from build123d import *

# Parameters (mm, degrees)
SKETCH_W        = 75
SKETCH_H        = 54
PAD_DEPTH       = 10
SKETCH001_R     = 17
POCKET_DEPTH    = 7
SKETCH002_W     = 111.709
SKETCH002_H     = 38.0948
POCKET001_DEPTH = 7
SKETCH003_R     = 2
POCKET002_DEPTH = 10.001
FILLET_R        = 10
CHAMFER_SIZE    = 0.5
CHAMFER001_SIZE = 1.5


with BuildPart() as part:
    # Sketch → Pad (new body)
    with BuildSketch(Plane.XY):
        with Locations((0, 7)):
            Rectangle(SKETCH_W, SKETCH_H)
    extrude(amount=PAD_DEPTH)

    # Sketch001 → Pocket (cut)
    with BuildSketch(Plane.XY.offset(10)):
        with Locations((-18, 0)):
            Circle(SKETCH001_R)
        with Locations((18, 0)):
            Circle(SKETCH001_R)
    extrude(amount=-POCKET_DEPTH, mode=Mode.SUBTRACT)

    # Sketch002 → Pocket001 (cut)
    with BuildSketch(Plane.XY.offset(10)):
        with Locations((0, 19.0474)):
            Rectangle(SKETCH002_W, SKETCH002_H)
    extrude(amount=-POCKET001_DEPTH, mode=Mode.SUBTRACT)

    # Sketch003 → Pocket002 (cut, through all)
    with BuildSketch(Plane.XY.offset(10)):
        with Locations((-18, 0)):
            Circle(SKETCH003_R)
        with Locations((18, 0)):
            Circle(SKETCH003_R)
    extrude(amount=-POCKET002_DEPTH, mode=Mode.SUBTRACT)

    # Fillet
    fillet_edges = [part.edges().sort_by_distance(p)[0] for p in [
        (37.5, 34, 1.5),
        (-37.5, 34, 1.5),
        (-37.5, -20, 5),
        (37.5, -20, 5),
    ]]
    fillet(fillet_edges, radius=FILLET_R)

    # Chamfer
    chamfer_edges = [part.edges().sort_by_distance(p)[0] for p in [
        (-37.5, -5, 10),
        (-34.571068, -17.071068, 10),
        (-36.25, 0, 10),
        (0, -20, 10),
        (-18, -17, 10),
        (34.571068, -17.071068, 10),
        (0, 0, 10),
        (37.5, -5, 10),
        (18, -17, 10),
        (36.25, 0, 10),
    ]]
    chamfer(chamfer_edges, length=CHAMFER_SIZE)

    # Chamfer001
    chamfer001_edges = [part.edges().sort_by_distance(p)[0] for p in [
        (18, -2, 3),
        (-18, -2, 3),
    ]]
    chamfer(chamfer001_edges, length=CHAMFER001_SIZE)


solid = part.part
Model file for the job. Use its own axes, mm. A direction names the side the tool comes from. Give positions to 0.01 mm unless a question says otherwise; leave off trailing zeros. Write each loop counter-clockwise with the first axis right and the second up, starting at its lowest first coordinate (ties: lowest second). Pieces come first, ordered by that corner, then holes. Notation, with made-up numbers: (6, 40.5) -> (61, 40.5) arc R21 cw to (61, 60.5) -> close; hole circle Ø10 at (28, 10). An arc over 180 degrees is marked (long way). Write item = value, one per line.
(1) Slice it at B-B, the plane x = 18. Give the cut face in (y, z), then the cut area to 4 significant figures.
Determined:
outline = (-20, 0) -> (-2, 0) -> (-2, 1.5) -> (-3.5, 3) -> (-17, 3) -> (-17, 9.5) -> (-17.5, 10) -> (-19.5, 10) -> (-20, 9.5) -> close; (2, 0) -> (34, 0) -> (34, 3) -> (3.5, 3) -> (2, 1.5) -> close
area = 168.5 mm2
(2) Flat gauge pins, fed straight in: P1, Ø12, axis at x = -13.5, y = 0.5, coming from the -Z side; P2, Ø2.5, axis at x = 18, y = 0, coming from the +Z side; P3, Ø6, axis at x = -10.5, y = 4.5, coming from the +Z side; P4, Ø4.5, axis at x = -18, y = 0, coming from the +Z side. Where does each tip first touch, or does it go through?
Determined:
P1 = 0
P2 = through
P3 = 3
P4 = 1.75
(3) Slice it at C-C, the plane z = 6.5. Give the cut face in (x, y), then the cut area to 3 significant figures.
Determined:
outline = (-37.5, -10) arc R10 ccw to (-27.5, -20) -> (27.5, -20) arc R10 ccw to (37.5, -10) -> (37.5, 0) -> (35, 0) arc R17 cw to (1, 0) -> (-1, 0) arc R17 cw to (-35, 0) -> (-37.5, 0) -> close
area = 549 mm2
(4) Mould opens along X. For faces 1 (the face through (-18, -17, 6)), 2 (the face through (0, -14, 10)), 3 (the face through (34.49, -17.15, 4.82)) say: released by +X, released by -X, zero draft, split by the parting line, or undercut.
Determined:
face_1 = undercut
face_2 = zero draft
face_3 = released by +X
(5) Tool access for faces 4 (the face through (-1, 9, 3)), 5 (the face through (0, 0, 6)), 6 (the face through (0, -20, 5)): list every direction of +Z, -Z, +X, -X, +Y, -Y with a clear straight run to the whole face (end or side of a thin tool).
Determined:
face_4 = +Z, +Y
face_5 = +Z, +X, -X, +Y
face_6 = +Z, -Z, +X, -X, -Y
(6) Probe line 1 along Y through (x, z) = (-18, 0.9); line 2 along X through (y, z) = (-9.5, 7); line 3 along Z through (x, y) = (22.5, 7). List the from-to ranges inside material, lowest first.
Determined:
line_1 = -20 to -2, 2 to 34
line_2 = -37.5 to -32.1, -3.9 to 3.9, 32.1 to 37.5
line_3 = 0 to 3
(7) Slice it at D-D, the plane y = 9. Give the cut face in (x, z), then the cut area to 3 significant figures.
Determined:
outline = (-37.5, 0) -> (37.5, 0) -> (37.5, 3) -> (-37.5, 3) -> close
area = 225 mm2
(8) Slice it at A-A, the plane z = 2.25. Give the cut face in (x, y), then the cut area to 3 significant figures.
Determined:
outline = (-37.5, -10) arc R10 ccw to (-27.5, -20) -> (27.5, -20) arc R10 ccw to (37.5, -10) -> (37.5, 24) arc R10 ccw to (27.5, 34) -> (-27.5, 34) arc R10 ccw to (-37.5, 24) -> close; hole circle Ø5.5 at (-18, 0); hole circle Ø5.5 at (18, 0)
area = 3,920 mm2
